Work out the finished part from the listing and answer in its coordinate system (mm). A direction names the side the tool comes from. Give positions to 0.01 mm unless a question says otherwise; leave off trailing zeros. Order: outer loops, then holes, each group sorted by start corner. A loop starts at its lowest first (then second) coordinate and runs counter-clockwise, first axis right, second up. Notation, with made-up numbers: M -27,28.5 L 31,28.5 A22 cw 31,62.5 Z; hole C 56.5,9.25 d1. An arc over 180 degrees is marked long. One line per item, written item: value.
from build123d import *

# Parameters (mm, degrees)
SKETCH_1_R      = 7.5
SKETCH_1_R_2    = 4
EXTRUDE_1_DEPTH = 24
CHAMFER_1_SIZE  = 0.5
SKETCH_2_W      = 0.35
SKETCH_2_H      = 1.1


with BuildPart() as part:
    # 草图1 → 凸台-拉伸1 (new body)
    with BuildSketch(Plane.XY):
        Circle(SKETCH_1_R)
        Circle(SKETCH_1_R_2, mode=Mode.SUBTRACT)
    extrude(amount=EXTRUDE_1_DEPTH)

    # 倒角1
    chamfer_1_edges = [part.edges().sort_by_distance(p)[0] for p in [
        (-7.5, 0, 0),
        (-7.5, 0, 24),
        (-4, 0, 0),
        (-4, 0, 24),
    ]]
    chamfer(chamfer_1_edges, length=CHAMFER_1_SIZE)

    # 草图2 → 切除-旋转1 (revolve, cut)
    with BuildSketch(Plane(origin=(0, 0, 0), x_dir=(1, 0, 0), z_dir=(0, 1, 0)), mode=Mode.PRIVATE) as cut_revolve_1_sk:
        with Locations((7.325, -3.8)):
            Rectangle(SKETCH_2_W, SKETCH_2_H)
        with Locations((7.325, -20.2)):
            Rectangle(SKETCH_2_W, SKETCH_2_H)
    revolve(cut_revolve_1_sk.sketch.rotate(Axis((0, 0, 0), (0, 0, 1)), 180), axis=Axis((0, 0, 0), (0, 0, 1)), mode=Mode.SUBTRACT)


solid = part.part
(1) Given P1, Ø5, axis at x = 4, z = 20, coming from the +Y side; P2, Ø8, axis at y = -5.5, z = 11, coming from the +X side, each flat-ended and moving along its own axis, determine where each tip first touches the part or whether it passes through.
Findings:
P1: stops at y = 7.34
P2: stops at x = 7.35
(2) Determine the mould class of faces 1 (the flat face through (0, -5, 24)), 2 (the cylindrical face through (-7.493, 0.33, 1.856)), 3 (the cylindrical face through (0.93, -7.09, 20.19)) for opening direction Z: pulls with the +Z half, pulls with the -Z half, needs draft (parallel to the pull), parting line crosses it, or undercut.
Findings:
face 1: pulls with the +Z half
face 2: needs draft
face 3: undercut
(3) Which of the six approach directions +Z, -Z, +X, -X, +Y, -Y give full straight-line access (tool end or side, diameter ignored) to faces 4 (the cylindrical face through (0.93, -7.09, 3.79)), 5 (the cylindrical face through (-0.867, -3.905, 11.839))?
Findings:
face 4: none
face 5: +Z, -Z
(4) Find the intervals of material crossed by probe 1 along Y at (x, z) = (0, 12.25); probe 2 along X at (y, z) = (3, 17.5); probe 3 along Y at (x, z) = (0.75, 23.25), in increasing order. Write a range as from..to.
Findings:
probe 1: y = -7.5..-4, 4..7.5
probe 2: x = -6.87..-2.65, 2.65..6.87
probe 3: y = -7.46..-3.93, 3.93..7.46
(5) Section C-C, the plane z = 11 is taken. Give the vertices of the cut face in (x, y), then the cut area to 3 significant figures.
Findings:
outline: C 0,0 d15; hole C 0,0 d8
area: 126 mm^2
